```python
from build123d import *

# Parameters (mm, degrees)
SKETCH1_R           = 4
SKETCH1_R_2         = 1.5
BOSS_EXTRUDE2_DEPTH = 4
SKETCH3_R           = 3.5
SKETCH3_R_2         = 2
CUT_EXTRUDE1_DEPTH  = 0.5
CUT_EXTRUDE2_START  = -0.5
SKETCH4_R           = 3.5
SKETCH4_R_2         = 2
CUT_EXTRUDE2_DEPTH  = 0.5


with BuildPart() as part:
    # Sketch1 → Boss-Extrude2 (new body)
    with BuildSketch(Plane.XY):
        Circle(SKETCH1_R)
        with Locations((0, 0.120165435)):
            Circle(SKETCH1_R_2, mode=Mode.SUBTRACT)
    extrude(amount=BOSS_EXTRUDE2_DEPTH)

    # Sketch3 → Cut-Extrude1 (cut)
    with BuildSketch(Plane.XY.offset(4)):
        Circle(SKETCH3_R)
        Circle(SKETCH3_R_2, mode=Mode.SUBTRACT)
    extrude(amount=-CUT_EXTRUDE1_DEPTH, mode=Mode.SUBTRACT)

    # Sketch4 → Cut-Extrude2 (cut)
    with BuildSketch(Plane(origin=(0, 0, 0), x_dir=(-1, 0, 0), z_dir=(0, 0, -1)).offset(CUT_EXTRUDE2_START)):
        with Locations(Location((0, 0, 0), (0, 0, 180))):
            Circle(SKETCH4_R)
        with Locations(Location((0, 0, 0), (0, 0, 180))):
            Circle(SKETCH4_R_2, mode=Mode.SUBTRACT)
    extrude(amount=CUT_EXTRUDE2_DEPTH, mode=Mode.SUBTRACT)


solid = part.part
```
Check sheet for the modelled part. Datum: model origin and axes. Units: mm. A direction names the side the tool comes from. Round coordinates to 2 decimals unless told otherwise and drop trailing zeros. Order: outer loops, then holes, each group sorted by start corner. A loop starts at its lowest first (then second) coordinate and runs counter-clockwise, first axis right, second up. Notation, with made-up numbers: (14.5, 66) - (55.5, 66) arc R7 ccw to (55.5, 71) - close; hole circle Ø1 at (26, -18). An arc over 180 degrees is marked (long way). Answer as CSV lines item,"result". Start each with the question number.
1) Tool access check on faces 4 (the face through (-0.434, -1.952, 3.754)), 5 (the face through (0.1, -1.6, 4)), 6 (the face through (3.233, 1.341, 0.254)). Record the directions out of +Z, -Z, +X, -X, +Y, -Y that give a thin tool (end or side, any length) a straight path to the whole face; none if there is none.
2) Section check D-D (y = -2.5). Record the cut outline in (x, z).
3) Section check A-A (x = 0). Record the cut outline in (y, z), then the cut area to 3 significant figures.
4) Section check C-C (x = 3). Record the cut outline in (y, z), then the cut area to 3 significant figures.
5) Depth check by flat-ended pin: pin 1 (1 mm diameter, centred on x = -2, y = 2, fed in from -Z). Enter the tip coordinate at first touch or a pass-through.
6) Section check B-B (y = 0). Record the cut outline in (x, z), then the cut area to 3 significant figures.
7) Draft check along Y on faces 1 (the face through (-1.5, 0.19, 1.97)), 2 (the face through (0.1, -1.6, 0)), 3 (the face through (-0.867, -3.905, 1.972)). Enter one of: +Y half, -Y half, draft (parallel to the pull), parting line (faces both ways), or undercut.
8) Scan lines: probe 1 along Y at (x, z) = (0, 3.75); probe 2 along Y at (x, z) = (0, 1.7); probe 3 along X at (y, z) = (-1.75, 3.7). Record each from-to range of solid material in increasing order.
Determined:
1,face 4,"+Z"
1,face 5,"+Z, +X, -X, +Y, -Y"
1,face 6,"-Z"
2,outline,"(-3.12, 0) - (-2.45, 0) - (-2.45, 0.5) - (2.45, 0.5) - (2.45, 0) - (3.12, 0) - (3.12, 4) - (2.45, 4) - (2.45, 3.5) - (-2.45, 3.5) - (-2.45, 4) - (-3.12, 4) - close"
3,outline,"(-4, 0) - (-3.5, 0) - (-3.5, 0.5) - (-2, 0.5) - (-2, 0) - (-1.38, 0) - (-1.38, 4) - (-2, 4) - (-2, 3.5) - (-3.5, 3.5) - (-3.5, 4) - (-4, 4) - close; (1.62, 0) - (2, 0) - (2, 0.5) - (3.5, 0.5) - (3.5, 0) - (4, 0) - (4, 4) - (3.5, 4) - (3.5, 3.5) - (2, 3.5) - (2, 4) - (1.62, 4) - close"
3,area,"17.0 mm^2"
4,outline,"(-2.65, 0) - (-1.8, 0) - (-1.8, 0.5) - (1.8, 0.5) - (1.8, 0) - (2.65, 0) - (2.65, 4) - (1.8, 4) - (1.8, 3.5) - (-1.8, 3.5) - (-1.8, 4) - (-2.65, 4) - close"
4,area,"17.6 mm^2"
5,pin 1,"z = 0.5"
6,outline,"(-4, 0) - (-3.5, 0) - (-3.5, 0.5) - (-2, 0.5) - (-2, 0) - (-1.5, 0) - (-1.5, 4) - (-2, 4) - (-2, 3.5) - (-3.5, 3.5) - (-3.5, 4) - (-4, 4) - close; (1.5, 0) - (2, 0) - (2, 0.5) - (3.5, 0.5) - (3.5, 0) - (4, 0) - (4, 4) - (3.5, 4) - (3.5, 3.5) - (2, 3.5) - (2, 4) - (1.5, 4) - close"
6,area,"17.0 mm^2"
7,face 1,"undercut"
7,face 2,"draft"
7,face 3,"parting line"
8,probe 1,"-4 to -3.5, -2 to -1.38, 1.62 to 2, 3.5 to 4"
8,probe 2,"-4 to -1.38, 1.62 to 4"
8,probe 3,"-3.6 to -3.03, -0.97 to 0.97, 3.03 to 3.6"
